Autodesk Inventor part; units mm, degrees
ref_plane "YZ Plane" through (0, 0, 0) normal (1, 0, 0) x (0, 1, 0)
ref_plane "XZ Plane" through (0, 0, 0) normal (0, 1, 0) x (-1, 0, 0)
ref_plane "XY Plane" through (0, 0, 0) normal (0, 0, 1) x (1, 0, 0)
sketch "Sketch3" plane through (0, 0, 0) normal (1, 0, 0) x (0, 1, 0)
  line L0 (0, 0) -> (76.2, 0)
  line L1 (76.2, 0) -> (76.2, -76.2)
  line L2 (76.2, -76.2) -> (0, -76.2)
  line L3 (0, -76.2) -> (0, 0)
  line L4 (76.2, 0) -> (50.8, 0)
  line L5 (50.8, 50.8) -> (76.2, 50.8)
  line L6 (76.2, 50.8) -> (76.2, 0)
  line L7 (76.2, -76.2) -> (50.8, -76.2)
  line L8 (50.8, -127) -> (76.2, -127)
  line L9 (76.2, -127) -> (76.2, -76.2)
  line L10 (50.8, 50.8) -> (-50.8, 50.8)
  line L11 (-50.8, 50.8) -> (-50.8, 0)
  line L12 (0, 0) -> (50.8, 0)
  line L13 (50.8, -76.2) -> (0, -76.2)
  line L14 (-50.8, -76.2) -> (-50.8, -127)
  line L15 (-50.8, -127) -> (50.8, -127)
  line L16 (0, 0) -> (0, -76.2)
  line L17 (-50.8, -76.2) -> (-50.8, 0)
  dimension "d1" = 76.2
  dimension "d26" = 50.8
extrude "Extrusion1" add sketch "Sketch3" along normal blind 25.4
sketch "Sketch5" plane through (0, 0, 0) normal (-1, 0, 0) x (0, 0, 1)
  line L0 (-76.2, 76.2) -> (0, 76.2)
  line L1 (-76.2, 76.2) -> (-38.1, 76.2)
  line L2 (-38.1, 76.2) -> (-38.1, 63.5)
  line L3 (-38.1, 63.5) -> (-38.1, 38.1)
  circle A0 centre (-38.1, 38.1) radius 11.2522
  point P0 (0, 0)
  dimension "d10" = 38.1
  dimension "d11" = 12.7
  dimension "d12" = 25.4
  dimension "d13" = 22.5044
extrude "Extrusion3" cut sketch "Sketch5" against normal blind 76.2
sketch "Sketch6" plane through (25.4, 0, 0) normal (1, 0, 0) x (0, 0, -1)
  circle A0 centre (38.1, 38.1) radius 11.2522
  circle A1 centre (38.1, 38.1) radius 19.05
  point P0 (0, 0)
  dimension "d20" = 38.1
extrude "Extrusion4" cut sketch "Sketch6" against normal blind 6.35
sketch "Sketch8" plane through (0, 76.2, 50.8) normal (0, 1, 0) x (1, 0, 0)
  line L0 (0, 0) -> (25.4, 0)
  line L1 (12.7, 0) -> (9.525, 0)
  line L2 (9.525, 0) -> (15.875, 0)
  line L3 (15.875, 0) -> (15.875, 50.8)
  line L4 (15.875, 50.8) -> (9.525, 50.8)
  line L5 (9.525, 50.8) -> (9.525, 0)
  line L6 (0, 177.8) -> (0, 0)
  line L7 (12.7, 177.8) -> (9.525, 177.8)
  line L8 (9.525, 177.8) -> (15.875, 177.8)
  line L9 (15.875, 177.8) -> (15.875, 127)
  line L10 (15.875, 127) -> (9.525, 127)
  line L11 (9.525, 127) -> (9.525, 177.8)
  line L12 (0, 0) -> (0, 177.8)
  point P0 (0, 50.8)
  point P1 (25.4, 177.8)
  point P2 (15.875, 0)
  dimension "d28" = 6.35
  dimension "d29" = 50.8
extrude "Extrusion5" cut sketch "Sketch8" against normal blind 76.2
sketch "Sketch9" plane through (0, -50.8, 50.8) normal (0, 0, 1) x (1, 0, 0)
  line L0 (9.525, 50.8) -> (15.875, 50.8)
  line L1 (15.875, 50.8) -> (15.875, 0)
  line L2 (15.875, 0) -> (9.525, 0)
  line L3 (9.525, 0) -> (9.525, 50.8)
  point P0 (0, 50.8)
  dimension "d32" = 6.35
  dimension "d33" = 50.8
extrude "Extrusion6" cut sketch "Sketch9" against normal blind 203.2
sketch "Sketch10" plane through (0, 0, 0) normal (-1, 0, 0) x (0, 0, 1)
  circle A0 centre (-38.1, 38.1) radius 11.2522
  circle A1 centre (-38.1, 38.1) radius 19.05
  point P0 (0, 0)
  dimension "d36" = 38.1
extrude "Extrusion7" cut sketch "Sketch10" against normal blind 5.08 contours A0 | A1
sketch "Sketch11" plane through (0, 76.2, 50.8) normal (0, 1, 0) x (1, 0, 0)
  line L0 (9.525, 50.8) -> (15.875, 50.8)
  line L1 (16.51, 50.8) -> (16.51, 0)
  line L2 (16.51, 0) -> (8.89, 0)
  line L3 (9.525, 177.8) -> (9.525, 0)
  line L4 (8.89, 0) -> (8.89, 51.308)
  line L5 (8.89, 0) -> (60.198, 0) construction
  line L6 (8.89, 51.308) -> (16.51, 51.308)
  line L7 (16.51, 51.308) -> (16.51, 50.8)
  line L8 (0, 69.85) -> (0, 107.95)
  line L9 (0, 88.9) -> (23.8125, 88.9)
  line L10 (9.525, 127) -> (15.875, 127)
  line L11 (16.51, 127) -> (16.51, 177.8)
  line L12 (16.51, 177.8) -> (8.89, 177.8)
  line L13 (8.89, 177.8) -> (8.89, 126.492)
  line L14 (8.89, 126.492) -> (16.51, 126.492)
  line L15 (16.51, 126.492) -> (16.51, 127)
  point P0 (0, 50.8)
  point P1 (0, 127)
  dimension "d40" = 7.62
extrude "Extrusion8" cut sketch "Sketch11" against normal blind 152.4
sketch "Sketch12" plane through (25.4, -50.8, 50.8) normal (0, 0, 1) x (1, 0, 0)
  line L0 (-8.89, 127) -> (-8.89, 0)
  line L1 (-16.51, 127) -> (-16.51, 0)
  line L2 (-8.89, 50.8) -> (-16.51, 50.8)
  line L3 (-16.51, 50.8) -> (-16.51, 0)
  line L4 (-16.51, 0) -> (-8.89, 0)
  line L5 (-8.89, 0) -> (-8.89, 50.8)
  point P0 (-25.4, 50.8)
extrude "Extrusion9" cut sketch "Sketch12" against normal blind 203.2
sketch "Sketch13" plane through (25.4, 0, 0) normal (1, 0, 0) x (0, 0, -1)
  line L0 (127, 76.2) -> (-50.8, 76.2)
  line L1 (-50.8, -50.8) -> (127, -50.8)
  line L2 (-50.8, 76.2) -> (-25.4, 76.2)
  line L3 (-25.4, 76.2) -> (-25.4, -50.8)
  line L4 (-25.4, -50.8) -> (-50.8, -50.8)
  line L5 (-50.8, -50.8) -> (-50.8, 76.2)
  line L6 (127, -50.8) -> (127, 76.2)
  line L7 (127, 76.2) -> (75.692, 76.2)
  line L8 (127, -50.8) -> (101.6, -50.8)
  line L9 (101.6, -50.8) -> (101.6, 76.2)
  line L10 (101.6, 76.2) -> (127, 76.2)
  line L11 (127, 76.2) -> (127, -50.8)
  point P0 (0, 0)
  dimension "d49" = 25.4
  dimension "d50" = 25.4
extrude "Extrusion10" cut sketch "Sketch13" against normal blind 25.4 contours L6 L1 L9 L0 | L3 L1 L5 L0
sketch "Sketch14" plane through (25.4, 0, 0) normal (1, 0, 0) x (0, 0, -1)
  line L0 (-25.4, -50.8) -> (101.6, -50.8)
  line L1 (101.6, -50.8) -> (101.6, 76.2)
  line L2 (-25.4, -50.8) -> (101.6, -50.8)
  line L3 (101.6, -50.8) -> (101.6, -12.7)
  line L4 (101.6, -12.7) -> (-25.4, -12.7)
  line L5 (-25.4, -12.7) -> (-25.4, -50.8)
  point P0 (0, 0)
  dimension "d53" = 38.1
extrude "Extrusion11" cut sketch "Sketch14" against normal blind 25.4
sketch "Sketch15" plane through (25.4, 0, 0) normal (1, 0, 0) x (0, 0, -1)
  point P0 (0, 0)
sketch "Sketch16" plane through (0, 76.2, 25.4) normal (0, 0, 1) x (1, 0, 0)
  point P0 (0, -76.2)
sketch "Sketch17" plane through (8.89, 76.2, -75.692) normal (0, 1, 0) x (1, 0, 0)
  line L0 (-8.89, -101.092) -> (0, -101.092)
  line L1 (7.62, 25.908) -> (7.62, -101.092)
  line L2 (0, -101.092) -> (7.62, -101.092)
  line L3 (7.62, -101.092) -> (7.62, -62.992)
  line L4 (7.62, -62.992) -> (0, -62.992)
  line L5 (0, -62.992) -> (0, -101.092)
  line L6 (7.62, 25.908) -> (7.62, 0)
  line L7 (0, -101.092) -> (0, 25.908)
  line L8 (7.62, 25.908) -> (0, 25.908)
  line L9 (0, 25.908) -> (0, -12.192)
  line L10 (0, -12.192) -> (7.62, -12.192)
  line L11 (7.62, -12.192) -> (7.62, 25.908)
  point P0 (-8.89, -75.692)
  point P1 (7.62, -12.192)
  dimension "d56" = 38.1
  dimension "d57" = 38.1
extrude "Extrusion12" cut sketch "Sketch17" against normal blind 76.2 contours L1 L10 L7 L8 | L1 L2 L5 L4
sketch "Sketch18" plane through (8.89, 0, -12.7) normal (0, -1, 0) x (1, 0, 0)
  point P0 (-8.89, 12.7)
sketch "Sketch19" plane through (25.4, 0, 0) normal (1, 0, 0) x (0, 0, -1)
  line L0 (12.7, 76.2) -> (-25.4, 76.2)
  line L1 (-25.4, -12.7) -> (-6.35, -12.7)
  line L2 (-6.35, -12.7) -> (-6.35, 76.2)
  line L3 (-6.35, 76.2) -> (-25.4, 76.2)
  line L4 (-25.4, 76.2) -> (-25.4, -12.7)
  line L5 (101.6, -12.7) -> (-25.4, -12.7)
  line L6 (101.6, 76.2) -> (-25.4, 76.2)
  line L7 (101.6, -12.7) -> (82.55, -12.7)
  line L8 (82.55, -12.7) -> (82.55, 76.2)
  line L9 (82.55, 76.2) -> (101.6, 76.2)
  line L10 (101.6, 76.2) -> (101.6, -12.7)
  point P0 (0, 0)
  dimension "d60" = 19.05
extrude "Extrusion13" cut sketch "Sketch19" against normal blind 76.2 contours L2 L1 L4 L0 | L6 L10 L5 L8
sketch "Sketch20" plane through (0, 76.2, 6.35) normal (0, 0, 1) x (1, 0, 0)
  line L0 (8.89, -88.9) -> (0, -88.9)
  line L1 (8.89, 0) -> (8.89, -76.2)
  line L2 (0, -88.9) -> (8.89, -88.9)
  line L3 (8.89, -88.9) -> (8.89, 0)
  line L4 (8.89, 0) -> (0, 0)
  line L5 (0, 0) -> (0, -88.9)
  point P0 (0, -76.2)
extrude "Extrusion14" cut sketch "Sketch20" against normal blind 127
sketch "Sketch21" plane through (25.4, 0, 0) normal (1, 0, 0) x (0, 0, -1)
  point P0 (0, 0)
sketch "Sketch22" plane through (16.51, 76.2, 6.35) normal (0, 1, 0) x (1, 0, 0)
  line L0 (0, 19.05) -> (-7.62, 19.05)
  line L1 (-7.62, 69.85) -> (0, 69.85)
  line L2 (0, 19.05) -> (-3.175, 19.05)
  line L3 (-3.175, 19.05) -> (-3.175, 69.85)
  line L4 (-3.175, 69.85) -> (0, 69.85)
  line L5 (0, 69.85) -> (0, 19.05)
  line L6 (-7.62, 69.85) -> (-7.62, 19.05)
  line L7 (-3.175, 69.85) -> (-7.62, 69.85)
  line L8 (-7.62, 69.85) -> (-7.62, 19.05)
  line L9 (-7.62, 19.05) -> (-3.175, 19.05)
  line L10 (-3.175, 19.05) -> (-3.175, 69.85)
  point P0 (-16.51, 6.35)
  point P1 (-3.175, 19.05)
  dimension "d65" = 3.175
extrude "Extrusion15" cut sketch "Sketch22" against normal blind 127 contours L0 L6 L1 L3
sketch "Sketch23" plane through (25.4, -12.7, 6.35) normal (0, 0, 1) x (1, 0, 0)
  line L0 (0, 88.9) -> (-8.89, 88.9)
  line L1 (-8.89, 0) -> (-2.54, 0)
  line L2 (-2.54, 0) -> (-2.54, 88.9)
  line L3 (-2.54, 88.9) -> (-8.89, 88.9)
  line L4 (-8.89, 88.9) -> (-8.89, 0)
  line L5 (-2.54, 88.9) -> (0, 88.9)
  line L6 (0, 88.9) -> (0, 0)
  line L7 (0, 0) -> (-2.54, 0)
  line L8 (-2.54, 0) -> (-2.54, 88.9)
  point P0 (-25.4, 12.7)
  dimension "d68" = 6.35
extrude "Extrusion16" cut sketch "Sketch23" against normal blind 127 contours L6 L7 L2 L0
sketch "Sketch24" plane through (22.86, -12.7, 6.35) normal (1, 0, 0) x (0, 0, -1)
  circle A0 centre (44.45, 50.8) radius 19.05
  circle A1 centre (44.45, 81.28) radius 3.175
  circle A2 centre (44.45, 20.32) radius 3.175
  point P0 (6.35, 12.7)
  dimension "d72" = 6.35
  dimension "d74" = 6.35
extrude "Extrusion17" cut sketch "Sketch24" against normal blind 127 contours A1 | A2
sketch "Sketch25" plane through (22.86, -12.7, 6.35) normal (1, 0, 0) x (0, 0, -1)
  circle A0 centre (44.45, 81.28) radius 3.175
  circle A1 centre (44.45, 81.28) radius 5.715
  circle A2 centre (44.45, 20.32) radius 3.175
  circle A3 centre (44.45, 20.32) radius 5.715
  point P0 (6.35, 12.7)
  dimension "d77" = 11.43
  dimension "d78" = 11.43
extrude "Extrusion18" cut sketch "Sketch25" against normal blind 5.08 contours A0 | A1 | A2 | A3
sketch "Sketch26" plane through (13.335, 76.2, -63.5) normal (-1, 0, 0) x (0, 0, 1)
  point P0 (63.5, -76.2)
sketch "Sketch27" plane through (22.86, -12.7, 6.35) normal (1, 0, 0) x (0, 0, -1)
  point P0 (6.35, 12.7)
sketch "Sketch28" plane through (13.335, 76.2, -63.5) normal (-1, 0, 0) x (0, 0, 1)
  point P0 (63.5, -76.2)
sketch "Sketch30" plane through (13.335, 76.2, -63.5) normal (-1, 0, 0) x (0, 0, 1)
  circle A0 centre (25.4, -7.62) radius 3.175
  circle A1 centre (25.4, -7.62) radius 3.175
  circle A2 centre (25.4, -38.1) radius 11.2522
  circle A3 centre (25.4, -38.1) radius 11.2522
  circle A4 centre (25.4, -68.58) radius 3.175
  circle A5 centre (25.4, -68.58) radius 3.175
  line L0 (0, -76.2) -> (50.8, -76.2)
  line L1 (50.8, -76.2) -> (50.8, 0)
  line L2 (50.8, 0) -> (0, 0)
  line L3 (0, 0) -> (0, -76.2)
  point P0 (63.5, -76.2)
extrude "Extrusion19" add sketch "Sketch30" along normal blind 0.635
properties part number "220307 Rod Support Part B Corrected"
Geometry check sheet. Reference: the model listing, model coordinates, mm. A direction names the side the tool comes from. Coordinates: 2 decimals unless noted, no trailing zeros. Order: outer loops, then holes, each group sorted by start corner. A loop starts at its lowest first (then second) coordinate and runs counter-clockwise, first axis right, second up. Notation, with made-up numbers: (1, -39) - (11, -39) arc R14 cw to (11, -14) - close; hole circle Ø8 at (29, 22). An arc over 180 degrees is marked (long way). Answer in a Markdown table with one row per item. Add a question column.
1) Cross-section at D-D, the plane z = -18. Record the cut outline in (x, y), then the cut area to 3 significant figures.
2) Cross-section at B-B, the plane y = 68.58. Record the cut outline in (x, z) (3 decimals), then the cut area to 3 significant figures.
3) Cross-section at A-A, the plane z = -38.1. State how many separate pieces and enclosed holes the cut face has, then the cut area to 3 significant figures.
4) Gauge pin test, flat ends, axial feed: P1, Ø1.1, axis at x = 14, z = -41, coming from the -Y side; P2, Ø1.1, axis at x = 14, y = 27.5, coming from the -Z side; P3, Ø2, axis at y = 39, z = -52.5, coming from the +X side. Record the tip position at first contact, or that the pin passes through.
5) Material ranges on line 1 along Y through (x, z) = (15.25, -38.1) (3 decimals); line 2 along Y through (x, z) = (16.65, -38.1) (3 decimals); line 3 along Z through (x, y) = (15.6, 7.62) (3 decimals), recorded low to high. Write a range as [from, to].
6) Set-up check for faces 1 (the flat face through (15, 0, -38)), 2 (the flat face through (17.78, 5, -41)), 3 (the flat face through (15, 39, -63.5)): record each of +Z, -Z, +X, -X, +Y, -Y from which the full face is reachable in a straight line by a thin tool's end or side.
7) Cross-section at C-C, the plane x = 21.5. Record the cut outline in (y, z) (3 decimals).
Check result:
| question | item | result |
|---|---|---|
| 1 | outline | (12.7, 0) - (16.51, 0) - (16.51, -12.7) - (22.86, -12.7) - (22.86, 76.2) - (12.7, 76.2) - close |
| 1 | area | 855 mm² |
| 2 | outline | (12.7, -63.5) - (16.51, -63.5) - (16.51, -82.55) - (22.86, -82.55) - (22.86, -43.815) - (17.78, -43.815) - (17.78, -41.275) - (12.7, -41.275) - close; (12.7, -34.925) - (17.78, -34.925) - (17.78, -32.385) - (22.86, -32.385) - (22.86, 6.35) - (16.51, 6.35) - (16.51, -12.7) - (12.7, -12.7) - close |
| 2 | area | 668 mm² |
| 3 | separate pieces | 4 |
| 3 | enclosed holes | 0 |
| 3 | area | 386 mm² |
| 4 | P1 | stops at y = 0 |
| 4 | P2 | stops at z = -63.5 |
| 4 | P3 | stops at x = 19.05 |
| 5 | line 1 | y = [0, 4.445], [10.795, 26.848], [49.352, 65.405], [71.755, 76.2] |
| 5 | line 2 | y = [-12.7, 4.445], [10.795, 26.848], [49.352, 65.405], [71.755, 76.2] |
| 5 | line 3 | z = [-63.5, -41.275], [-34.925, -12.7] |
| 6 | face 1 | +Z, -Z, -X, -Y |
| 6 | face 2 | +X |
| 6 | face 3 | -Z, -X, +Y, -Y |
| 7 | outline | (-12.7, -82.55) - (76.2, -82.55) - (76.2, 6.35) - (-12.7, 6.35) - close; hole circle Ø11.43 at (7.62, -38.1); hole circle Ø38.1 at (38.1, -38.1); hole circle Ø11.43 at (68.58, -38.1) |
